For this review, take the finished solid that the model builds, in its own axes (mm). A direction names the side the tool comes from. Give positions to 0.01 mm unless a question says otherwise; leave off trailing zeros. Order: outer loops, then holes, each group sorted by start corner. A loop starts at its lowest first (then second) coordinate and runs counter-clockwise, first axis right, second up. Notation, with made-up numbers: (-21, -16) - (21, -16) arc R6 ccw to (21, -9) - close; hole circle Ø4 at (72.5, 42.5). An arc over 180 degrees is marked (long way). Use a Markdown table: item, result. Add a question column.
1) We need section B-B on y = 15.24. Write out the cut boundary in (x, z) (3 decimals), then the cut area to 3 significant figures.
2) We need section D-D on z = 6.75. Write out the cut boundary in (x, y) (3 decimals), then the cut area to 3 significant figures.
3) Wall thickness on L1, parallel to Y at x = 91.25, z = 19.05 (3 decimals); L2, parallel to X at y = 17.5, z = 19.05; L3, parallel to X at y = 9.5, z = 19.05: over which ranges is each line inside the solid? List them lowest first.
4) We need section C-C on x = 12.7. Write out the cut boundary in (y, z) (3 decimals), then the cut area to 3 significant figures.
5) We need section A-A on x = 84.5. Write out the cut boundary in (y, z) (3 decimals).
6) Mouldability with a two-part tool opening along X and no side actions: class faces 5 (the face through (14.25, 15.34, 17.02)), 6 (the face through (51, 2.54, 2)), 7 (the face through (95.25, 4, 16)) as released by +X, released by -X, zero draft, split by the parting line, or undercut.
7) Machinability: for faces 1 (the face through (86, 20.955, 20)), 2 (the face through (88.811, 24.193, 17.233)), 3 (the face through (95.25, 27, 16)), 4 (the face through (51.42, 15.52, 15.87)), which of the approach directions +Z, -Z, +X, -X, +Y, -Y give a long, thin tool a straight path to every point of the face, cutting with its end or side? Answer none if there is none.
8) Clearance check with flat-ended pins moving along their axes: P1, Ø3, axis at x = 69.85, z = 19.05, coming from the -Y side; P2, Ø12.5, axis at y = 16, z = 5.5, coming from the +X side; P3, Ø3, axis at y = 17.5, z = 18.5, coming from the +X side; P4, Ø3.5, axis at y = 24.765, z = 19.05, coming from the +X side. State where each tip first meets the part, or that it passes through.
Autodesk Inventor part; units mm, degrees
ref_plane "YZ Plane" through (0, 0, 0) normal (1, 0, 0) x (0, 1, 0)
ref_plane "XZ Plane" through (0, 0, 0) normal (0, 1, 0) x (-1, 0, 0)
ref_plane "XY Plane" through (0, 0, 0) normal (0, 0, 1) x (1, 0, 0)
sketch "Sketch1" plane through (0, 0, 0) normal (1, 0, 0) x (0, 1, 0)
  line L0 (0, 0) -> (31.115, 0)
  line L1 (31.115, 0) -> (31.115, 25.4)
  line L2 (31.115, 25.4) -> (0, 25.4)
  line L3 (0, 25.4) -> (0, 0)
  dimension "d0" = 25.4
  dimension "d1" = 31.115
extrude "Extrusion1" add sketch "Sketch1" along normal blind 95.25
sketch "Sketch2" plane through (95.25, 0, 0) normal (1, 0, 0) x (0, 0, -1)
  arc A0 (-3.175, 27.94) -> (-3.175, 2.54) centre (-3.175, 15.24) ccw
  line L0 (0, 0) -> (0, 31.115)
  line L1 (-25.4, 0) -> (0, 0)
  line L2 (-3.175, 27.94) -> (0, 27.94)
  line L3 (-3.175, 2.54) -> (0, 2.54)
  dimension "d4" = 3.175
  dimension "d5" = 15.24
  dimension "d6" = 25.4
extrude "Extrusion2" cut sketch "Sketch2" against normal blind 88.9
sketch "Sketch3" plane through (0, 31.115, 25.4) normal (0, 1, 0) x (1, 0, 0)
  line L0 (0, 25.4) -> (0, 0)
  line L1 (95.25, 25.4) -> (95.25, 0)
  line L2 (0, 0) -> (95.25, 0)
  point P0 (12.7, 6.35)
  point P1 (69.85, 6.35)
  dimension "d9" = 0
  dimension "d10" = 12.7
  dimension "d12" = 6.35
  dimension "d35" = 69.85
hole "Hole1" at (12.7, 31.115, 19.05) at (69.85, 31.115, 19.05) direction (0, -1, 0) diameter 5.1054 end through all
sketch "Sketch5" plane through (95.25, 0, 0) normal (1, 0, 0) x (0, 0, -1)
  line L0 (-25.4, 31.115) -> (-25.4, 0)
  line L1 (-25.4, 0) -> (0, 0)
  line L2 (-25.4, 31.115) -> (-25.4, 0)
  line L3 (0, 31.115) -> (-25.4, 31.115)
  point P0 (-19.05, 24.765)
  point P1 (-19.05, 6.35)
  point P2 (-25.4, 10.16)
  point P3 (-25.4, 20.32)
  dimension "d24" = 6.35
  dimension "d25" = 6.35
  dimension "d26" = 6.35
  dimension "d27" = 6.35
hole "Hole2" at (95.25, 24.765, 19.05) at (95.25, 6.35, 19.05) direction (-1, 0, 0) diameter 3.81 depth 12.7 tip angle 118.188
sketch "Sketch6" plane through (95.25, 0, 0) normal (1, 0, 0) x (0, 0, -1)
  line L0 (-38.1122, 20.955) -> (-10.5779, 20.955)
  line L1 (-10.5779, 20.955) -> (-10.5779, 10.16)
  line L2 (-10.5779, 10.16) -> (-38.1122, 10.16)
  line L3 (-38.1122, 10.16) -> (-38.1122, 20.955)
  line L4 (-25.4, 0) -> (0, 0)
  line L5 (0, 31.115) -> (-25.4, 31.115)
  dimension "d36" = 10.16
  dimension "d37" = 10.16
extrude "Extrusion4" cut sketch "Sketch6" against normal blind 19.05
properties part number "BatteryRail"
Checked values:
| question | item | result |
|---|---|---|
| 1 | outline | (0, 0) - (6.35, 0) - (6.35, 15.875) - (76.2, 15.875) - (76.2, 25.4) - (0, 25.4) - close; hole circle Ø5.105 at (12.7, 19.05); hole circle Ø5.105 at (69.85, 19.05) |
| 1 | area | 786 mm² |
| 2 | outline | (0, 0) - (95.25, 0) - (95.25, 3.054) - (6.35, 3.054) - (6.35, 27.426) - (95.25, 27.426) - (95.25, 31.115) - (0, 31.115) - close |
| 2 | area | 797 mm² |
| 3 | L1 | 0 to 4.445, 8.255 to 10.16, 20.955 to 22.86, 26.67 to 31.115 |
| 3 | L2 | 0 to 10.15, 15.25 to 67.3, 72.4 to 76.2 |
| 3 | L3 | 0 to 10.15, 15.25 to 67.3, 72.4 to 95.25 |
| 4 | outline | (0, 0) - (2.54, 0) - (2.54, 3.175) arc R12.7 cw to (27.94, 3.175) - (27.94, 0) - (31.115, 0) - (31.115, 16.497) - (0, 16.497) - close; (0, 21.603) - (31.115, 21.603) - (31.115, 25.4) - (0, 25.4) - close |
| 4 | area | 297 mm² |
| 5 | outline | (0, 0) - (2.54, 0) - (2.54, 3.175) arc R12.7 cw to (10.16, 14.815) - (10.16, 25.4) - (0, 25.4) - close; (20.955, 14.516) arc R12.7 cw to (27.94, 3.175) - (27.94, 0) - (31.115, 0) - (31.115, 25.4) - (20.955, 25.4) - close; hole circle Ø3.81 at (6.35, 19.05); hole circle Ø3.81 at (24.765, 19.05) |
| 6 | face 5 | undercut |
| 6 | face 6 | zero draft |
| 6 | face 7 | released by +X |
| 7 | face 1 | +Z, -Z, +X |
| 7 | face 2 | +X |
| 7 | face 3 | +Z, -Z, +X, +Y, -Y |
| 7 | face 4 | -Z, +X |
| 8 | P1 | through |
| 8 | P2 | x = 6.35 |
| 8 | P3 | x = 76.2 |
| 8 | P4 | x = 82.46 |
